The figure shows three views and two pictorial views of one solid part (mm, origin at its lowest corner). Answer the questions. Coordinates: 2 decimals unless noted, no trailing zeros. Loops run counter-clockwise (first coordinate to the right, second up) from the corner with the lowest first, then second, coordinate; pieces in that order, holes last. Notation, with made-up numbers: M -36,46.25 L -1,46.25 A29 cw -1,72.25 Z; hole C -33,85.5 d5. An arc over 180 degrees is marked long. One line per item, written item: value. Start each with the question number.
1. Consider probe 1 along Y at (x, z) = (215.5, 23.5); probe 2 along X at (y, z) = (195.5, 29); probe 3 along Z at (x, y) = (72.5, 215). Determine where each line is inside the solid, lowest interval first.
2. Flat-ended cylindrical pins translate along their axes: pin 1 (8 mm diameter, centred on x = 93.5, y = 100.5, fed in from -Z); pin 2 (8 mm diameter, centred on y = 156.5, z = 23, fed in from -X); pin 3 (5 mm diameter, centred on x = 58.5, y = 165, fed in from +Z); pin 4 (12 mm diameter, centred on x = 138.5, y = 137.5, fed in from +Z). Find the tip coordinate at first contact, or state that the pin passes through.
3. The part is cut by section B-B (y = 165). Write down the section's boundary in (x, z).
4. The part is cut by section C-C (x = 56.65). Write down the section's boundary in (y, z).
5. The part is cut by section D-D (z = 37). Write down the section's boundary in (x, y).
6. The part is cut by section A-A (x = 205.5). Write down the section's boundary in (y, z).
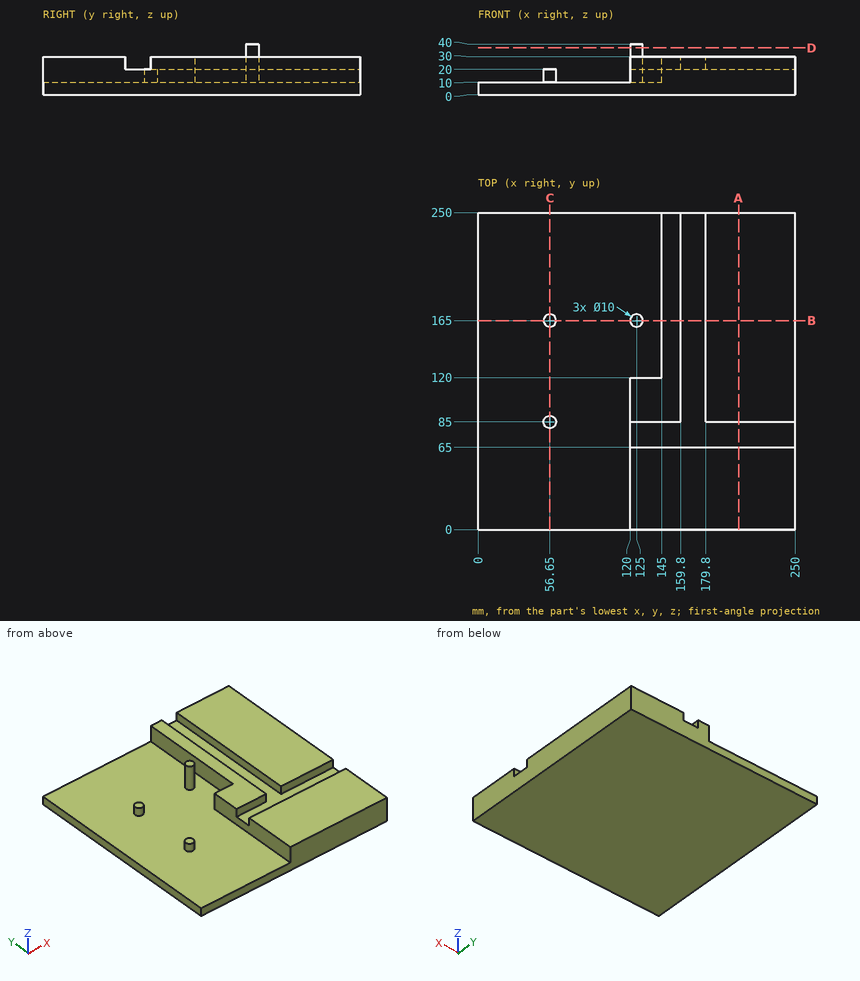
Answer block:
1. probe 1: y = 0 to 65, 85 to 250
1. probe 2: x = 145 to 159.8, 179.8 to 250
1. probe 3: z = 0 to 10
2. pin 1: stops at z = 0
2. pin 2: stops at x = 122.82
2. pin 3: stops at z = 20
2. pin 4: stops at z = 10
3. outline: M 0,0 L 250,0 L 250,30 L 179.8,30 L 179.8,20 L 159.8,20 L 159.8,30 L 145,30 L 145,10 L 130,10 L 130,40 L 120,40 L 120,10 L 61.65,10 L 61.65,20 L 51.65,20 L 51.65,10 L 0,10 Z
4. outline: M 0,0 L 250,0 L 250,10 L 170,10 L 170,20 L 160,20 L 160,10 L 90,10 L 90,20 L 80,20 L 80,10 L 0,10 Z
5. outline: C 125,165 d10
6. outline: M 0,0 L 250,0 L 250,30 L 85,30 L 85,20 L 65,20 L 65,30 L 0,30 Z
